```python
from build123d import *

# Parameters (mm, degrees)
CUT_EXTRUDE1_START  = -27
SKETCH6_R           = 1.75
CUT_EXTRUDE1_DEPTH  = 5.7500001
SKETCH7_R           = 5.05
BOSS_EXTRUDE2_DEPTH = 8
FILLET1_R           = 2
SKETCH8_R           = 2.5
BOSS_EXTRUDE3_DEPTH = 25.4


with BuildPart() as part:
    # Sketch3 → Revolve1 (revolve)
    with BuildSketch(Plane(origin=(0, 0, 0), x_dir=(1, 0, 0), z_dir=(0, 1, 0))):
        with BuildLine():
            Line((0, 25.32), (27.625, 25.32))
            Line((27.625, 25.32), (27.625, 26.5))
            ThreePointArc((27.625, 26.5), (27.917893219, 27.207106781), (28.625, 27.5))
            Line((28.625, 27.5), (30.75, 27.5))
            ThreePointArc((30.75, 27.5), (31.457106781, 27.207106781), (31.75, 26.5))
            Line((31.75, 26.5), (31.75, -7.5))
            add(Edge.make_bspline(
                [(0, -28.5), (23.295574904, -28.5), (31.75, -20.206509843), (31.75, -7.5)],
                knots=[0, 0, 0, 0, 1, 1, 1, 1], degree=3))
            Line((0, -28.5), (0, 25.32))
        make_face()
    revolve(axis=Axis((0, 0, -65.333333333), (0, 0, 1)))

    # Sketch6 → Cut-Extrude1 (cut, through all)
    with BuildSketch(Plane(origin=(0, 0, 0), x_dir=(1, 0, 0), z_dir=(0, 1, 0)).offset(CUT_EXTRUDE1_START)):
        Circle(SKETCH6_R)
    cut_extrude1 = extrude(amount=-CUT_EXTRUDE1_DEPTH, mode=Mode.SUBTRACT)

    # Mirror1: Cut-Extrude1 across plane
    add(cut_extrude1.mirror(Plane.ZX), mode=Mode.SUBTRACT)

    # Sketch7 → Boss-Extrude2 (add)
    with BuildSketch(Plane.XY.offset(25)):
        Circle(SKETCH7_R)
    extrude(amount=BOSS_EXTRUDE2_DEPTH)

    # Fillet1
    fillet1_edges = [part.edges().sort_by_distance(p)[0] for p in [
        (-5.05, 0, 33),
    ]]
    fillet(fillet1_edges, radius=FILLET1_R)

    # Sketch8 → Boss-Extrude3 (add)
    with BuildSketch(Plane.XY.offset(33)):
        Circle(SKETCH8_R)
    extrude(amount=BOSS_EXTRUDE3_DEPTH)


solid = part.part
```
Design review of the part built by this model. Coordinates are the model's own, in mm. A direction names the side the tool comes from. Coordinates: 2 decimals unless noted, no trailing zeros. Loops run counter-clockwise (first coordinate to the right, second up) from the corner with the lowest first, then second, coordinate; pieces in that order, holes last.
Q1. Tool access review of faces 1 (the face through (0, 27, 0)), 2 (the face through (0, 0, -25.32)), 3 (the face through (0, -27, 0)), 4 (the face through (-0.54, -2.44, 45.52)): name each direction out of +Z, -Z, +X, -X, +Y, -Y from which nothing blocks a thin tool from reaching the whole face with its end or side.
Reported:
face 1: +Y
face 2: -Z
face 3: -Y
face 4: +Z
Q2. We need section B-B on z = 47.5. State the section outline as (x, y) points, and give its area (3 significant figures).
Reported:
outline: circle Ø5 at (0, 0)
area: 19.6 mm2
Q3. To check wall thickness, follow line 1 (Y direction, x = 0, z = -26.3) (3 decimals); line 2 (X direction, y = 29.05, z = 0); line 3 (Y direction, x = 26, z = 14). State the ranges of each line that lie inside material, in increasing order.
Reported:
line 1: y = -31.75 to -27.625, 27.625 to 31.75
line 2: x = -12.81 to -1.75, 1.75 to 12.81
line 3: y = -16.63 to 16.63
Q4. For pin 1 (6 mm diameter, centred on y = -12.5, z = 0.5, fed in from +X); pin 2 (1 mm diameter, centred on x = -0.5, z = 0.5, fed in from -Y); pin 3 (1.5 mm diameter, centred on y = 7, z = 7, fed in from +X), all flat-tipped, find the tip position at first contact; note any pin that passes through.
Reported:
pin 1: stops at x = 30.3
pin 2: stops at y = -27
pin 3: stops at x = 31.13
Q5. We need section A-A on z = 0. State the section outline as (x, y) points, and give its area (3 significant figures).
Reported:
outline: (-1.75, -31.7) - (-1.75, -27) - (1.75, -27) - (1.75, -31.7) arc R31.75 ccw to (1.75, 31.7) - (1.75, 27) - (-1.75, 27) - (-1.75, 31.7) arc R31.75 ccw to start
area: 3,130 mm2
Q6. The part is to be moulded in two halves that separate along Y. For faces 5 (the face through (1.617, -29.343, 0.67)), 6 (the face through (-5.989, -26.968, -25.918)), 7 (the face through (4.817, 1.517, 29.661)), say which applies: +Y half, -Y half, draft (parallel to the pull), parting line (faces both ways), or undercut.
Reported:
face 5: draft
face 6: undercut
face 7: parting line
